Verification items for the finished model (mm, model axes). Give positions to 0.01 mm unless a question says otherwise; leave off trailing zeros. Loops run counter-clockwise (first coordinate to the right, second up) from the corner with the lowest first, then second, coordinate; pieces in that order, holes last. Notation, with made-up numbers: M 3,21 L 22,21 A10 cw 22,35 Z; hole C 64,82.25 d10. An arc over 180 degrees is marked long. Use a Markdown table: item, result.
from build123d import *

# Parameters (mm, degrees)
BOSS_EXTRUDE1_DEPTH = 1219.2
SKETCH3_W           = 1219.2
SKETCH3_H           = 6.35
BOSS_EXTRUDE2_DEPTH = 1.778
SKETCH4_W           = 1219.2
SKETCH4_H           = 6.35
BOSS_EXTRUDE3_DEPTH = 1.778
FILLET1_R           = 5.08
SHELL1_START        = 2.54
SHELL1_DEPTH        = 1214.12
CUT_EXTRUDE1_REACH  = 1222.671
SKETCH6_W           = 25.4
SKETCH6_H           = 25.4
SKETCH7_R           = 15.875
SKETCH7_R_2         = 12.7
BOSS_EXTRUDE4_DEPTH = 25.4
CUT_EXTRUDE2_REACH  = 1222.256
SKETCH10_R          = 12.7
BOSS_EXTRUDE5_START = 25.4
SKETCH11_R          = 15.875
SKETCH11_R_2        = 12.7
BOSS_EXTRUDE5_DEPTH = 25.4
CUT_EXTRUDE3_REACH  = 1247.634
SKETCH12_R          = 12.7


# Read off the part's stored shape, not the designer's step: Shell1
with BuildPart() as part:
    # Sketch1 → Boss-Extrude1 (new body)
    with BuildSketch(Plane.XY):
        Polygon((-44.45, -17.145), (-44.45, 17.145), (44.45, 17.145), (44.45, -17.145), (0, -20.955), align=None)
    extrude(amount=BOSS_EXTRUDE1_DEPTH)

    # Sketch3 → Boss-Extrude2 (add)
    with BuildSketch(Plane.ZY.offset(44.45)):
        with Locations((609.6, 13.97)):
            Rectangle(SKETCH3_W, SKETCH3_H)
    extrude(amount=BOSS_EXTRUDE2_DEPTH)

    # Sketch4 → Boss-Extrude3 (add)
    with BuildSketch(Plane(origin=(44.45, 0, 0), x_dir=(0, 0, -1), z_dir=(1, 0, 0))):
        with Locations((-609.6, 13.97)):
            Rectangle(SKETCH4_W, SKETCH4_H)
    extrude(amount=BOSS_EXTRUDE3_DEPTH)

    # Fillet1
    fillet1_edges = [part.edges().sort_by_distance(p)[0] for p in [
        (44.45, -17.145, 609.6),
        (-44.45, -17.145, 609.6),
    ]]
    fillet(fillet1_edges, radius=FILLET1_R)

    # Shell1 outline → Shell1 (cut)
    with BuildSketch(Plane.XY.offset(SHELL1_START)):
        with BuildLine():
            Line((41.91, -12.481801497), (41.91, 13.335))
            Line((41.91, 13.335), (43.688, 13.335))
            Line((43.688, 13.335), (43.688, 14.605))
            Line((43.688, 14.605), (-43.688, 14.605))
            Line((-43.688, 14.605), (-43.688, 13.335))
            Line((-43.688, 13.335), (-41.91, 13.335))
            Line((-41.91, 13.335), (-41.91, -12.481801497))
            ThreePointArc((-41.91, -12.481801497), (-41.241172627, -14.199449016), (-39.586918899, -15.012521986))
            Line((-39.586918899, -15.012521986), (0, -18.405686463))
            Line((0, -18.405686463), (39.586918899, -15.012521986))
            ThreePointArc((39.586918899, -15.012521986), (41.241172627, -14.199449016), (41.91, -12.481801497))
        make_face()
    extrude(amount=SHELL1_DEPTH, mode=Mode.SUBTRACT)

    # Sketch6 → Cut-Extrude1 (cut, up to next)
    with BuildSketch(Plane(origin=(0, 17.145, 0), x_dir=(1, 0, 0), z_dir=(0, 1, 0)), mode=Mode.PRIVATE) as cut_extrude1_sk1:
        with Locations((0, -1155.7)):
            Rectangle(SKETCH6_W, SKETCH6_H)
    cut_extrude1_tool1 = extrude(cut_extrude1_sk1.sketch, amount=-CUT_EXTRUDE1_REACH, mode=Mode.PRIVATE) & part.part
    # Sketch6 → Cut-Extrude1 (cut, up to next)
    with BuildSketch(Plane(origin=(0, 17.145, 0), x_dir=(1, 0, 0), z_dir=(0, 1, 0)), mode=Mode.PRIVATE) as cut_extrude1_sk2:
        with Locations((0, -952.5)):
            Rectangle(SKETCH6_W, SKETCH6_H)
    cut_extrude1_tool2 = extrude(cut_extrude1_sk2.sketch, amount=-CUT_EXTRUDE1_REACH, mode=Mode.PRIVATE) & part.part
    # Sketch6 → Cut-Extrude1 (cut, up to next)
    with BuildSketch(Plane(origin=(0, 17.145, 0), x_dir=(1, 0, 0), z_dir=(0, 1, 0)), mode=Mode.PRIVATE) as cut_extrude1_sk3:
        with Locations((0, -749.3)):
            Rectangle(SKETCH6_W, SKETCH6_H)
    cut_extrude1_tool3 = extrude(cut_extrude1_sk3.sketch, amount=-CUT_EXTRUDE1_REACH, mode=Mode.PRIVATE) & part.part
    # Sketch6 → Cut-Extrude1 (cut, up to next)
    with BuildSketch(Plane(origin=(0, 17.145, 0), x_dir=(1, 0, 0), z_dir=(0, 1, 0)), mode=Mode.PRIVATE) as cut_extrude1_sk4:
        with Locations((0, -546.1)):
            Rectangle(SKETCH6_W, SKETCH6_H)
    cut_extrude1_tool4 = extrude(cut_extrude1_sk4.sketch, amount=-CUT_EXTRUDE1_REACH, mode=Mode.PRIVATE) & part.part
    # Sketch6 → Cut-Extrude1 (cut, up to next)
    with BuildSketch(Plane(origin=(0, 17.145, 0), x_dir=(1, 0, 0), z_dir=(0, 1, 0)), mode=Mode.PRIVATE) as cut_extrude1_sk5:
        with Locations((0, -342.9)):
            Rectangle(SKETCH6_W, SKETCH6_H)
    cut_extrude1_tool5 = extrude(cut_extrude1_sk5.sketch, amount=-CUT_EXTRUDE1_REACH, mode=Mode.PRIVATE) & part.part
    # Sketch6 → Cut-Extrude1 (cut, up to next)
    with BuildSketch(Plane(origin=(0, 17.145, 0), x_dir=(1, 0, 0), z_dir=(0, 1, 0)), mode=Mode.PRIVATE) as cut_extrude1_sk6:
        with Locations((0, -139.7)):
            Rectangle(SKETCH6_W, SKETCH6_H)
    cut_extrude1_tool6 = extrude(cut_extrude1_sk6.sketch, amount=-CUT_EXTRUDE1_REACH, mode=Mode.PRIVATE) & part.part
    add(cut_extrude1_tool1.solids().sort_by_distance((0, 17.145, 1155.7))[0], mode=Mode.SUBTRACT)
    add(cut_extrude1_tool2.solids().sort_by_distance((0, 17.145, 952.5))[0], mode=Mode.SUBTRACT)
    add(cut_extrude1_tool3.solids().sort_by_distance((0, 17.145, 749.3))[0], mode=Mode.SUBTRACT)
    add(cut_extrude1_tool4.solids().sort_by_distance((0, 17.145, 546.1))[0], mode=Mode.SUBTRACT)
    add(cut_extrude1_tool5.solids().sort_by_distance((0, 17.145, 342.9))[0], mode=Mode.SUBTRACT)
    add(cut_extrude1_tool6.solids().sort_by_distance((0, 17.145, 139.7))[0], mode=Mode.SUBTRACT)

    # Sketch7 → Boss-Extrude4 (add)
    with BuildSketch(Plane(origin=(0, 0, 0), x_dir=(-1, 0, 0), z_dir=(0, 0, -1))):
        with Locations(Location((0, -5.08, 0), (0, 0, 260.201815092))):
            Circle(SKETCH7_R)
        with Locations((0, -5.08)):
            Circle(SKETCH7_R_2, mode=Mode.SUBTRACT)
    extrude(amount=BOSS_EXTRUDE4_DEPTH)

    # Sketch10 → Cut-Extrude2 (cut, up to next)
    with BuildSketch(Plane(origin=(0, 0, 0), x_dir=(-1, 0, 0), z_dir=(0, 0, -1)), mode=Mode.PRIVATE) as cut_extrude2_sk1:
        with Locations((0, -5.08)):
            Circle(SKETCH10_R)
    cut_extrude2_tool1 = extrude(cut_extrude2_sk1.sketch, amount=-CUT_EXTRUDE2_REACH, mode=Mode.PRIVATE) & part.part
    add(cut_extrude2_tool1.solids().sort_by_distance((0, -5.08, 0))[0], mode=Mode.SUBTRACT)

    # Sketch11 → Boss-Extrude5 (add)
    with BuildSketch(Plane.XY.offset(1219.2).offset(BOSS_EXTRUDE5_START)):
        with Locations(Location((0, -5.08, 0), (0, 0, 279.798184908))):
            Circle(SKETCH11_R)
        with Locations(Location((0, -5.08, 0), (0, 0, 180))):
            Circle(SKETCH11_R_2, mode=Mode.SUBTRACT)
    extrude(amount=-BOSS_EXTRUDE5_DEPTH)

    # Sketch12 → Cut-Extrude3 (cut, up to next)
    with BuildSketch(Plane.XY.offset(1219.2), mode=Mode.PRIVATE) as cut_extrude3_sk1:
        with Locations(Location((0, -5.08, 0), (0, 0, 180))):
            Circle(SKETCH12_R)
    cut_extrude3_tool1 = extrude(cut_extrude3_sk1.sketch, amount=-CUT_EXTRUDE3_REACH, mode=Mode.PRIVATE) & part.part
    add(cut_extrude3_tool1.solids().sort_by_distance((0, -5.08, 1219.2))[0], mode=Mode.SUBTRACT)


solid = part.part
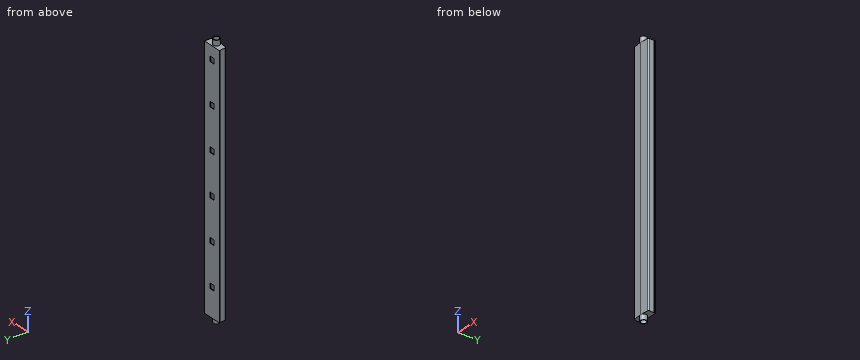
(1) Gauge pin test, flat ends, axial feed: P1, Ø3, axis at x = 0.5, y = 15.5, coming from the +Z side; P2, Ø0.8, axis at x = -6, y = 16.5, coming from the -Z side; P3, Ø12, axis at x = 10, z = 941, coming from the +Y side (3 decimals); P4, Ø1.5, axis at y = 5, z = 1057, coming from the -X side. Record the tip position at first contact, or that the pin passes through.
Results below:
| item | result |
|---|---|
| P1 | z = 1219.2 |
| P2 | z = 0 |
| P3 | y = 17.145 |
| P4 | x = -44.45 |
(2) Cross-section at A-A on y = -5.08. Record the cut outline in (x, z) (3 decimals).
Results below:
| item | result |
|---|---|
| outline | M -44.45,0 L -15.875,0 L -15.875,-25.4 L -12.7,-25.4 L -12.7,2.54 L -41.91,2.54 L -41.91,1216.66 L -12.7,1216.66 L -12.7,1244.6 L -15.875,1244.6 L -15.875,1219.2 L -44.45,1219.2 Z; M 12.7,-25.4 L 15.875,-25.4 L 15.875,0 L 44.45,0 L 44.45,1219.2 L 15.875,1219.2 L 15.875,1244.6 L 12.7,1244.6 L 12.7,1216.66 L 41.91,1216.66 L 41.91,2.54 L 12.7,2.54 Z |
(3) Cross-section at C-C on x = -29. Record the cut outline in (y, z) (3 decimals).
Results below:
| item | result |
|---|---|
| outline | M -18.469,0 L 17.145,0 L 17.145,1219.2 L -18.469,1219.2 Z; hole M -15.92,2.54 L 14.605,2.54 L 14.605,1216.66 L -15.92,1216.66 Z |
(4) Cross-section at B-B on z = 695. Record the cut outline in (x, y) (3 decimals), then the cut area to 3 significant figures.
Results below:
| item | result |
|---|---|
| outline | M -46.228,10.795 L -44.45,10.795 L -44.45,-12.482 A5.08 ccw -39.804,-17.543 L 0,-20.955 L 39.804,-17.543 A5.08 ccw 44.45,-12.482 L 44.45,10.795 L 46.228,10.795 L 46.228,17.145 L -46.228,17.145 Z; hole M -43.688,13.335 L -41.91,13.335 L -41.91,-12.482 A2.54 ccw -39.587,-15.013 L 0,-18.406 L 39.587,-15.013 A2.54 ccw 41.91,-12.482 L 41.91,13.335 L 43.688,13.335 L 43.688,14.605 L -43.688,14.605 Z |
| area | 613 mm^2 |
(5) Material ranges on line 1 (X direction, y = -7, z = 1182.5); line 2 (Z direction, x = 32, y = 12); line 3 (Z direction, x = -12, y = 5), recorded low to high.
Results below:
| item | result |
|---|---|
| line 1 | -44.45 to -41.91, 41.91 to 44.45 |
| line 2 | 0 to 2.54, 1216.66 to 1219.2 |
| line 3 | -25.4 to 2.54, 1216.66 to 1244.6 |
